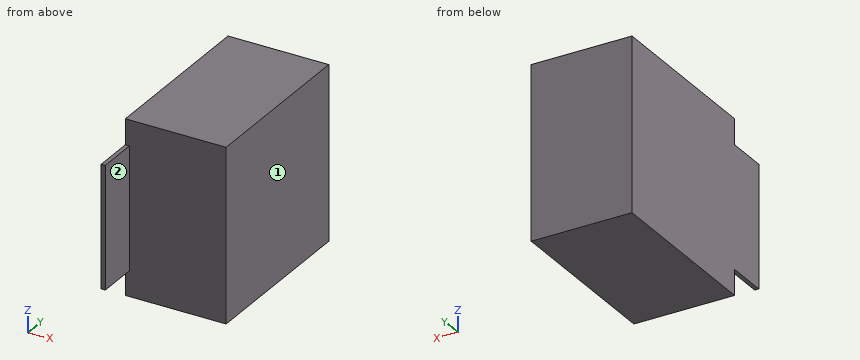
Autodesk Inventor part; units mm, degrees
ref_plane "YZ Plane" through (0, 0, 0) normal (1, 0, 0) x (0, 1, 0)
ref_plane "XZ Plane" through (0, 0, 0) normal (0, 1, 0) x (-1, 0, 0)
ref_plane "XY Plane" through (0, 0, 0) normal (0, 0, 1) x (1, 0, 0)
sketch "Эскиз1" plane through (0, 0, 0) normal (1, 0, 0) x (0, 1, 0)
  line L0 (-4.25, 4.25) -> (4.25, 4.25)
  line L1 (4.25, 4.25) -> (4.25, -4.25)
  line L2 (4.25, -4.25) -> (-4.25, -4.25)
  line L3 (-4.25, -4.25) -> (-4.25, 4.25)
  line L4 (-4.25, 4.25) -> (4.25, -4.25) construction
  line L5 (4.25, 4.25) -> (-4.25, -4.25) construction
  point P0 (0, 0)
  dimension "d0" = 8.5
  dimension "d1" = 8.5
extrude "Выдавливание1" add sketch "Эскиз1" along normal blind 4.95
sketch "Эскиз2" plane through (0, -4.25, -4.25) normal (0, -1, 0) x (1, 0, 0)
  line L0 (0.2, 7.25) -> (0, 7.25)
  line L1 (0, 7.25) -> (0, 1.25)
  line L2 (0, 1.25) -> (0.2, 1.25)
  line L3 (0.2, 1.25) -> (0.2, 7.25)
  line L4 (0.2, 7.25) -> (0, 1.25) construction
  line L5 (0, 7.25) -> (0.2, 1.25) construction
  line L6 (0, 8.5) -> (0, 0)
  point P0 (0, 4.25)
  point P1 (0.1, 4.25)
  point P2 (0, 4.25)
  dimension "d4" = 0.2
  dimension "d5" = 6
extrude "Выдавливание2" add sketch "Эскиз2" along normal blind 2
properties part number "camera"
Model file for the job. Use its own axes, mm. Face numbers are marked on the shaded views. A direction names the side the tool comes from. Give positions to 0.01 mm unless a question says otherwise; leave off trailing zeros. Order: outer loops, then holes, each group sorted by start corner. A loop starts at its lowest first (then second) coordinate and runs counter-clockwise, first axis right, second up. Notation, with made-up numbers: (73, -29.5) - (98, -29.5) arc R28 cw to (98, -4.5) - close; hole circle Ø3 at (70, -12). An arc over 180 degrees is marked (long way). One line per item, written item: value.
Item 1: Slice it at B-B (x = 4.55). List the corners of the cut face in (y, z).
Response values:
outline: (-4.25, -4.25) - (4.25, -4.25) - (4.25, 4.25) - (-4.25, 4.25) - close
Item 2: Tool access for the marked faces 1 and 2: list every direction of +Z, -Z, +X, -X, +Y, -Y with a clear straight run to the whole face (end or side of a thin tool).
Response values:
face 1: +Z, -Z, +X, +Y, -Y
face 2: +Z, -Z, +X, -Y
Item 3: Wall check: line 1 (Y direction, x = 0.65, z = 1); line 2 (X direction, y = -5.25, z = -2). Give the ranges that are in metal, low to high.
Response values:
line 1: -4.25 to 4.25
line 2: 0 to 0.2
Item 4: Slice it at C-C (z = 3.5). List the corners of the cut face in (x, y), then the cut area to 3 significant figures.
Response values:
outline: (0, -4.25) - (4.95, -4.25) - (4.95, 4.25) - (0, 4.25) - close
area: 42.1 mm2
Item 5: Pin check, flat tips, straight feed: pin 1 Ø2 at (x, y) = (2.5, -5) entering from +Z; pin 2 Ø0.6 at (y, z) = (-5, 1) entering from +X. Stop position of each tip, or through.
Response values:
pin 1: z = 4.25
pin 2: x = 0.2
Item 6: Slice it at A-A (z = -1.5). List the corners of the cut face in (x, y).
Response values:
outline: (0, -6.25) - (0.2, -6.25) - (0.2, -4.25) - (4.95, -4.25) - (4.95, 4.25) - (0, 4.25) - close
